Build history of the part. All positions in model axes, mm. A direction names the side the tool comes from. Give positions to 0.01 mm unless a question says otherwise; leave off trailing zeros. Loops run counter-clockwise (first coordinate to the right, second up) from the corner with the lowest first, then second, coordinate; pieces in that order, holes last.
1) Band-saw the part on C-C on x = 36. List the corners of the cut face in (y, z).
2) Band-saw the part on B-B on z = 3.15. State how many separate pieces and enclosed holes the cut face has, then the cut area to 3 significant figures.
3) Flat gauge pin, fed straight in: P1, Ø2, axis at x = 23.5, z = 2, coming from the -Y side. Where does the tip first touch, or does it go through?
4) Band-saw the part on D-D on x = 22.5. List the corners of the cut face in (y, z), then the cut area to 3 significant figures.
5) 3-axis set-ups, long thin cutter, end or side, ignore diameter. For faces 5 (the flat face through (23, -5.155, 2)), 6 (the flat face through (13, -1.106, 2)), 7 (the flat face through (42.775, -4.353, 1.972)): which of +Z, -Z, +X, -X, +Y, -Y reach the whole face in a straight line?
6) Wall check: line 1 (Y direction, x = 18.5, z = 1.4); line 2 (X direction, y = -1, z = 1); line 3 (Y direction, x = 20, z = 1.7). Give the ranges that are in metal, low to high.
7) Band-saw the part on A-A on x = 15. List the corners of the cut face in (y, z).
8) Two-plate mould, pull along X, no slides. Class faces 1 (the cylindrical face through (3.005, -0.042, 1.972)), 2 (the cylindrical face through (56.39, 3.31, 1.97)), 3 (the cylindrical face through (-0.245, 0.002, 1.972)), 4 (the cylindrical face through (10.82, -6.98, 1.97)): +X half, -X half, draft (parallel to the pull), parting line (faces both ways), or undercut.
```python
from build123d import *

# Parameters (mm, degrees)
SKETCH1_R           = 0.75
SKETCH1_R_2         = 1.25
SKETCH1_R_3         = 1
BOSS_EXTRUDE1_DEPTH = 4


with BuildPart() as part:
    # Sketch1 → Boss-Extrude1 (new body)
    with BuildSketch(Plane.XY):
        with BuildLine():
            ThreePointArc((46.980351469, -3.99295605), (47.960883487, -3.859840066), (48.923458954, -3.63046837))
            Line((48.923458954, -3.63046837), (58.781132355, 1.635320677))
            ThreePointArc((58.781132355, 1.635320677), (56.34843078, 3.327817207), (53.445513313, 3.924182561))
            Line((53.445513313, 3.924182561), (4.34174303, 4.401750396))
            Line((4.34174303, 4.401750396), (4.254220138, 4.402601616))
            ThreePointArc((4.254220138, 4.402601616), (-0.245779862, -0.097398384), (4.254220138, -4.597398384))
            Line((4.254220138, -4.597398384), (8.346946684, -5.15524466))
            Line((8.346946684, -5.15524466), (8.439838836, -5.15524466))
            ThreePointArc((8.439838836, -5.15524466), (10.866040294, -6.980836707), (13.292241752, -5.15524466))
            Line((13.292241752, -5.15524466), (24.292241752, -5.15524466))
            Line((24.292241752, -5.15524466), (32.304248164, -5.15524466))
            ThreePointArc((32.304248164, -5.15524466), (35.607637679, -6.523335594), (38.685278543, -4.70339554))
            Line((38.685278543, -4.70339554), (46.980351469, -3.99295605))
        make_face()
        with Locations((10.866040294, -4.455836707)):
            Circle(SKETCH1_R, mode=Mode.SUBTRACT)
        with BuildLine():
            ThreePointArc((9.719017648, -2.106433547), (9.219017648, -1.606433547), (9.719017648, -1.106433547))
            Line((9.719017648, -1.106433547), (17.146734956, -1.106433547))
            Line((17.146734956, -1.106433547), (16.355916602, -1.897251901))
            Line((16.355916602, -1.897251901), (9.750504349, -2.10544115))
            ThreePointArc((9.750504349, -2.10544115), (9.734768816, -2.106185386), (9.719017648, -2.106433547))
        make_face(mode=Mode.SUBTRACT)
        with Locations((35.325099909, -2.10544115)):
            Circle(SKETCH1_R_2, mode=Mode.SUBTRACT)
        with Locations((4.254220138, -0.097398384)):
            Circle(SKETCH1_R_2, mode=Mode.SUBTRACT)
        with Locations((54.495894224, 1.635320677)):
            Circle(SKETCH1_R_3, mode=Mode.SUBTRACT)
    extrude(amount=BOSS_EXTRUDE1_DEPTH)


solid = part.part
```
Findings below:
1. outline: (-6.48, 0) - (-3.16, 0) - (-3.16, 4) - (-6.48, 4) - close; (-1.05, 0) - (4.09, 0) - (4.09, 4) - (-1.05, 4) - close
2. separate pieces: 1
2. enclosed holes: 5
2. area: 474 mm2
3. P1: stops at y = -5.16
4. outline: (-5.16, 0) - (4.23, 0) - (4.23, 4) - (-5.16, 4) - close
4. area: 37.5 mm2
5. face 5: +Z, -Z, -Y
5. face 6: +Z, -Z
5. face 7: +Z, -Z, +X, -Y
6. line 1: y = -5.16 to 4.26
6. line 2: x = -0.15 to 3.39, 5.12 to 34.74, 35.91 to 53.85
6. line 3: y = -5.16 to 4.25
7. outline: (-5.16, 0) - (-1.94, 0) - (-1.94, 4) - (-5.16, 4) - close; (-1.11, 0) - (4.3, 0) - (4.3, 4) - (-1.11, 4) - close
8. face 1: undercut
8. face 2: +X half
8. face 3: -X half
8. face 4: undercut
